Check sheet for the modelled part. Datum: model origin and axes. Units: mm. A direction names the side the tool comes from. Give positions to 0.01 mm unless a question says otherwise; leave off trailing zeros. Write each loop counter-clockwise with the first axis right and the second up, starting at its lowest first coordinate (ties: lowest second). Pieces come first, ordered by that corner, then holes. Notation, with made-up numbers: M -29,49.5 L -4,49.5 A5 ccw -4,54.5 Z; hole C -12.5,54.5 d3. An arc over 180 degrees is marked long. Use CSV: the item, a comma, the result in double quotes. Start each with the question number.
1. Cross-section at D-D, the plane x = -32.5. Enter the section's corners in (y, z), and give its area (3 significant figures).
2. Depth check by flat-ended pin: P1, Ø8, axis at x = -19, y = 3, coming from the +Z side; P2, Ø3, axis at x = -21, y = 2, coming from the +Z side; P3, Ø2.5, axis at x = -31.66, y = 3.3, coming from the -Z side; P4, Ø5, axis at x = -6.5, y = 1.5, coming from the -Z side. Enter the tip coordinate at first touch or a pass-through.
3. Cross-section at C-C, the plane z = -16.25. Enter the section's corners in (x, y).
4. Cross-section at B-B, the plane y = 2. State how many separate pieces and enclosed holes the cut face has, and give its area (3 significant figures).
5. Mould release check, pull along X, two halves, no side actions. Record for faces 1 (the face through (0.345, 3, -13)), 2 (the face through (-5, 8.301, -13)), 3 (the face through (-33.76, 3.21, -12.72)): +X half, -X half, draft (parallel to the pull), parting line (faces both ways), or undercut.
6. Cross-section at A-A, the plane z = -13.75. Enter the section's corners in (x, y), and give its area (3 significant figures).
7. Scan lines: line 1 (X direction, y = 1.5, z = -13); line 2 (Z direction, x = -31.5, y = 0.5); line 3 (X direction, y = 5, z = -13.75). Record each from-to range of solid material in increasing order.
8. Access from +Z, -Z, +X, -X, +Y, -Y to the whole of each face (thin tool, end or side, straight path). Record for faces 4 (the face through (-16.3, 10.301, -18.3)), 5 (the face through (-6, 4, -14.196)), 6 (the face through (-29, 3, -14.196)).
from build123d import *

# Parameters (mm, degrees)
PAD037_DEPTH      = 13
PAD037_DEPTH_BACK = 1
SKETCH058_W       = 1.93
SKETCH058_H       = 10
PAD038_DEPTH      = 3
SKETCH059_W       = 10
SKETCH059_H       = 3
PAD039_DEPTH      = 9
SKETCH060_W       = 10
SKETCH060_H       = 3
PAD040_DEPTH      = 9
SKETCH070_R       = 2.1
HOLE_DEPTH        = 3.001
FILLET014_R       = 0.5


with BuildPart() as part:
    # Sketch057 (on Face1 of CopyPad023) → Pad037 (new body, two sides)
    with BuildSketch(Plane(origin=(0, -35.363644, -2), x_dir=(1, 0, 0), z_dir=(0, -1, 0))) as pad037_sk:
        with BuildLine():
            ThreePointArc((-25.035308, -10.895555), (-17.960308, -17.970555), (-10.885308, -10.895554))
            Line((-10.885308, -10.895554), (-8.960308, -10.895554))
            ThreePointArc((-26.960308, -10.895555), (-17.960308, -19.895555), (-8.960308, -10.895554))
            Line((-26.960308, -10.895555), (-25.035308, -10.895555))
        make_face()
    extrude(amount=-PAD037_DEPTH)
    extrude(pad037_sk.sketch, amount=PAD037_DEPTH_BACK)

    # Sketch058 (on Face1 of Pad037) → Pad038 (join)
    with BuildSketch(Plane.XY.offset(-12.895555)):
        with Locations((-25.995308, -29.363644)):
            Rectangle(SKETCH058_W, SKETCH058_H)
        with Locations((-9.920308, -29.363644)):
            Rectangle(SKETCH058_W, SKETCH058_H)
    extrude(amount=-PAD038_DEPTH)

    # Sketch059 (on Face12 of Pad038) → Pad039 (join)
    with BuildSketch(Plane(origin=(-26.960308, 0, -2), x_dir=(0, -1, 0), z_dir=(-1, 0, 0))):
        with Locations((29.363644, -12.395555)):
            Rectangle(SKETCH059_W, SKETCH059_H)
    extrude(amount=PAD039_DEPTH)

    # Sketch060 (on Face13 of Pad039) → Pad040 (join)
    with BuildSketch(Plane(origin=(-8.955308, 0, -2), x_dir=(0, 1, 0), z_dir=(1, 0, 0))):
        with Locations((-29.363644, -12.395555)):
            Rectangle(SKETCH060_W, SKETCH060_H)
    extrude(amount=PAD040_DEPTH)

    # Sketch070 (on Face15 of Pad040) → Hole (cut, through all)
    with BuildSketch(Plane(origin=(0, 0, -15.895555), x_dir=(1, 0, 0), z_dir=(0, 0, -1))):
        with Locations((-31.960308, 29.363644)):
            Circle(SKETCH070_R)
        with Locations((-3.955308, 29.363644)):
            Circle(SKETCH070_R)
    extrude(amount=-HOLE_DEPTH, mode=Mode.SUBTRACT)

    # Fillet014
    fillet014_edges = [part.edges().sort_by_distance(p)[0] for p in [
        (-35.960308, -24.363644, -14.395555),
        (-35.960308, -34.363644, -14.395555),
        (0.044692, -24.363644, -14.395555),
        (0.044692, -34.363644, -14.395555),
    ]]
    fillet(fillet014_edges, radius=FILLET014_R)


with BuildPart() as part_1:
    # Body007 placement: moved
    add(part.part.moved(Location((0.3, 32.66415, 1.7))))


solid = part_1.part
Worked answers:
1,outline,"M -1.7,-14.2 L 1.38,-14.2 L 1.38,-11.2 L -1.7,-11.2 Z; M 5.23,-14.2 L 8.3,-14.2 L 8.3,-11.2 L 5.23,-11.2 Z"
1,area,"18.5 mm^2"
2,P1,"stops at z = -15.84"
2,P2,"stops at z = -16.36"
2,P3,"passes through"
2,P4,"stops at z = -14.2"
3,outline,"M -25.11,-3.7 L -22.61,-3.7 L -22.61,10.3 L -25.11,10.3 Z; M -12.71,-3.7 L -10.21,-3.7 L -10.21,10.3 L -12.71,10.3 Z"
4,separate pieces,"3"
4,enclosed holes,"0"
4,area,"83.9 mm^2"
5,face 1,"+X half"
5,face 2,"draft"
5,face 3,"undercut"
6,outline,"M -35.66,-1.2 A0.5 ccw -35.16,-1.7 L -26.29,-1.7 L -26.29,-3.7 L -24.26,-3.7 L -24.26,10.3 L -26.29,10.3 L -26.29,8.3 L -35.16,8.3 A0.5 ccw -35.66,7.8 Z; M -11.06,-3.7 L -9.03,-3.7 L -9.03,-1.7 L -0.16,-1.7 A0.5 ccw 0.34,-1.2 L 0.34,7.8 A0.5 ccw -0.16,8.3 L -9.03,8.3 L -9.03,10.3 L -11.06,10.3 Z; hole C -31.66,3.3 d4.2; hole C -3.66,3.3 d4.2"
6,area,"216 mm^2"
7,line 1,"x = -35.66 to -32.74, -30.58 to -24.5, -10.82 to -4.74, -2.57 to 0.34"
7,line 2,"z = -14.2 to -11.2"
7,line 3,"x = -35.66 to -32.89, -30.43 to -24.26, -11.06 to -4.89, -2.42 to 0.34"
8,face 4,"+Z, -Z, +X, -X, +Y"
8,face 5,"-Z, +X, +Y, -Y"
8,face 6,"-Z, -X, +Y, -Y"
